Can you work these out from the model? Positions are in its coordinate system, mm. A direction names the side the tool comes from. Round coordinates to 2 decimals unless told otherwise and drop trailing zeros. Loops run counter-clockwise (first coordinate to the right, second up) from the corner with the lowest first, then second, coordinate; pieces in that order, holes last. Notation, with made-up numbers: (-31, 10.25) -> (-8, 10.25) arc R4 ccw to (-8, 15.25) -> close; hole circle Ø4 at (-10, 42). An arc over 180 degrees is marked (long way). Use a Markdown table: item, result.
from build123d import *

# Parameters (mm, degrees)
SKETCH1_W           = 381
SKETCH1_H           = 50.8
BOSS_EXTRUDE1_DEPTH = 2.794
SKETCH2_W           = 381
SKETCH2_H           = 2.794
BOSS_EXTRUDE2_DEPTH = 48.006
SKETCH3_R           = 3.429
SKETCH3_R_2         = 3.3734375
CUT_EXTRUDE1_DEPTH  = 2.794


with BuildPart() as part:
    # Sketch1 → Boss-Extrude1 (new body)
    with BuildSketch(Plane(origin=(0, 0, 0), x_dir=(1, 0, 0), z_dir=(0, 1, 0))):
        Rectangle(SKETCH1_W, SKETCH1_H)
    extrude(amount=BOSS_EXTRUDE1_DEPTH)

    # Sketch2 → Boss-Extrude2 (add)
    with BuildSketch(Plane(origin=(0, 2.794, 0), x_dir=(1, 0, 0), z_dir=(0, 1, 0))):
        with Locations((0, -24.003)):
            Rectangle(SKETCH2_W, SKETCH2_H)
    extrude(amount=BOSS_EXTRUDE2_DEPTH)

    # Sketch3 → Cut-Extrude1 (cut)
    with BuildSketch(Plane.XY.offset(25.4)):
        with Locations((0, 38.1)):
            Circle(SKETCH3_R)
        with Locations((0, 12.7)):
            Circle(SKETCH3_R_2)
    extrude(amount=-CUT_EXTRUDE1_DEPTH, mode=Mode.SUBTRACT)


solid = part.part
1. Which directions (+Z, -Z, +X, -X, +Y, -Y) give clear straight access to the entire face, cutting with the end or side of a thin tool? Please do faces 4 (the flat face through (-3, 0, 0)), 5 (the flat face through (-3, 26, 22.606)).
Answer sheet:
| item | result |
|---|---|
| face 4 | +Z, -Z, +X, -X, -Y |
| face 5 | -Z, +X, -X, +Y |
2. I want a section at C-C (z = 13). Please give me the cut outline in (x, y).
Answer sheet:
| item | result |
|---|---|
| outline | (-190.5, 0) -> (190.5, 0) -> (190.5, 2.79) -> (-190.5, 2.79) -> close |
3. I want a section at D-D (y = 38.1). Please give me the cut outline in (x, z).
Answer sheet:
| item | result |
|---|---|
| outline | (-190.5, 22.61) -> (-3.43, 22.61) -> (-3.43, 25.4) -> (-190.5, 25.4) -> close; (3.43, 22.61) -> (190.5, 22.61) -> (190.5, 25.4) -> (3.43, 25.4) -> close |
4. Will these pins go through, and if not, where does the flat tip stop? pin 1 Ø10 at (x, z) = (-119.5, 11.5) entering from +Y; pin 2 Ø24 at (x, y) = (-78.5, 34) entering from -Z.
Answer sheet:
| item | result |
|---|---|
| pin 1 | stops at y = 2.79 |
| pin 2 | stops at z = 22.61 |
5. I want a section at B-B (y = 12.7). Please give me the cut outline in (x, z).
Answer sheet:
| item | result |
|---|---|
| outline | (-190.5, 22.61) -> (-3.37, 22.61) -> (-3.37, 25.4) -> (-190.5, 25.4) -> close; (3.37, 22.61) -> (190.5, 22.61) -> (190.5, 25.4) -> (3.37, 25.4) -> close |
6. I want a section at A-A (x = 0). Please give me the cut outline in (y, z), plus the area to 3 significant figures.
Answer sheet:
| item | result |
|---|---|
| outline | (0, -25.4) -> (2.79, -25.4) -> (2.79, 22.61) -> (9.33, 22.61) -> (9.33, 25.4) -> (0, 25.4) -> close; (16.07, 22.61) -> (34.67, 22.61) -> (34.67, 25.4) -> (16.07, 25.4) -> close; (41.53, 22.61) -> (50.8, 22.61) -> (50.8, 25.4) -> (41.53, 25.4) -> close |
| area | 238 mm² |
7. If we mould it in two halves opening along X, with no side actions, what happens to faces 1 (the flat face through (190.5, 14, 23)), 2 (the flat face through (-3, 2.794, -2)), 3 (the cylindrical face through (-0.45, 41.5, 24.02))? For each: +X half, -X half, draft (parallel to the pull), parting line (faces both ways), or undercut.
Answer sheet:
| item | result |
|---|---|
| face 1 | +X half |
| face 2 | draft |
| face 3 | undercut |
8. I need wall thicknesses on line 1 (Y direction, x = 0, z = 23); line 2 (X direction, y = 12, z = 23); line 3 (X direction, y = 38, z = 24). Which ranges of each line are inside material? Lowest first, please.
Answer sheet:
| item | result |
|---|---|
| line 1 | y = 0 to 9.33, 16.07 to 34.67, 41.53 to 50.8 |
| line 2 | x = -190.5 to -3.3, 3.3 to 190.5 |
| line 3 | x = -190.5 to -3.43, 3.43 to 190.5 |
